Verification items for this drawing (mm, ordinates from the low corner). A direction names the side the tool comes from. Round coordinates to 2 decimals unless told otherwise and drop trailing zeros. Write each loop counter-clockwise with the first axis right and the second up, starting at its lowest first coordinate (ties: lowest second). Pieces come first, ordered by that corner, then holes. Notation, with made-up numbers: M 72,3.5 L 98,3.5 A31 cw 98,41.5 Z; hole C 57.5,3.5 d1. An arc over 180 degrees is marked long. One line per question, with ' | ' between items. Start each with the question number.
Q1. Tool access check on the marked faces 1, 2 and 3. Record the directions out of +Z, -Z, +X, -X, +Y, -Y that give a thin tool (end or side, any length) a straight path to the whole face; none if there is none.
Q2. Gauge pin test, flat ends, axial feed: pin 1 (3 mm diameter, centred on x = 41, y = 21, fed in from -Z); pin 2 (5 mm diameter, centred on x = 32.5, z = 35, fed in from -Y); pin 3 (12 mm diameter, centred on y = 32, z = 68, fed in from -X) (1 decimal). Record the tip position at first contact, or that the pin passes through.
Q3. Cross-section at B-B (y = 29). Record the boundary of the cut face in (x, z) (1 decimal).
Q4. Thickness scan on line 1 along X through (y, z) = (32, 61.5) (1 decimal); line 2 along Y through (x, z) = (65.5, 50.5); line 3 along X through (y, z) = (10.5, 40) (1 decimal). Record the ranges inside material, lowest first. Write a range as from..to.
Q5. Cross-section at A-A (y = 24). Record the boundary of the cut face in (x, z) (1 decimal).
Q6. Release check for a two-part mould opening along Z. For the marked faces 4, 5, 6 and 7 record: released by +Z, released by -Z, zero draft, split by the parting line, or undercut.
Q7. Cross-section at C-C (y = 4.5). Record the boundary of the cut face in (x, z), then the cut area to 3 significant figures.
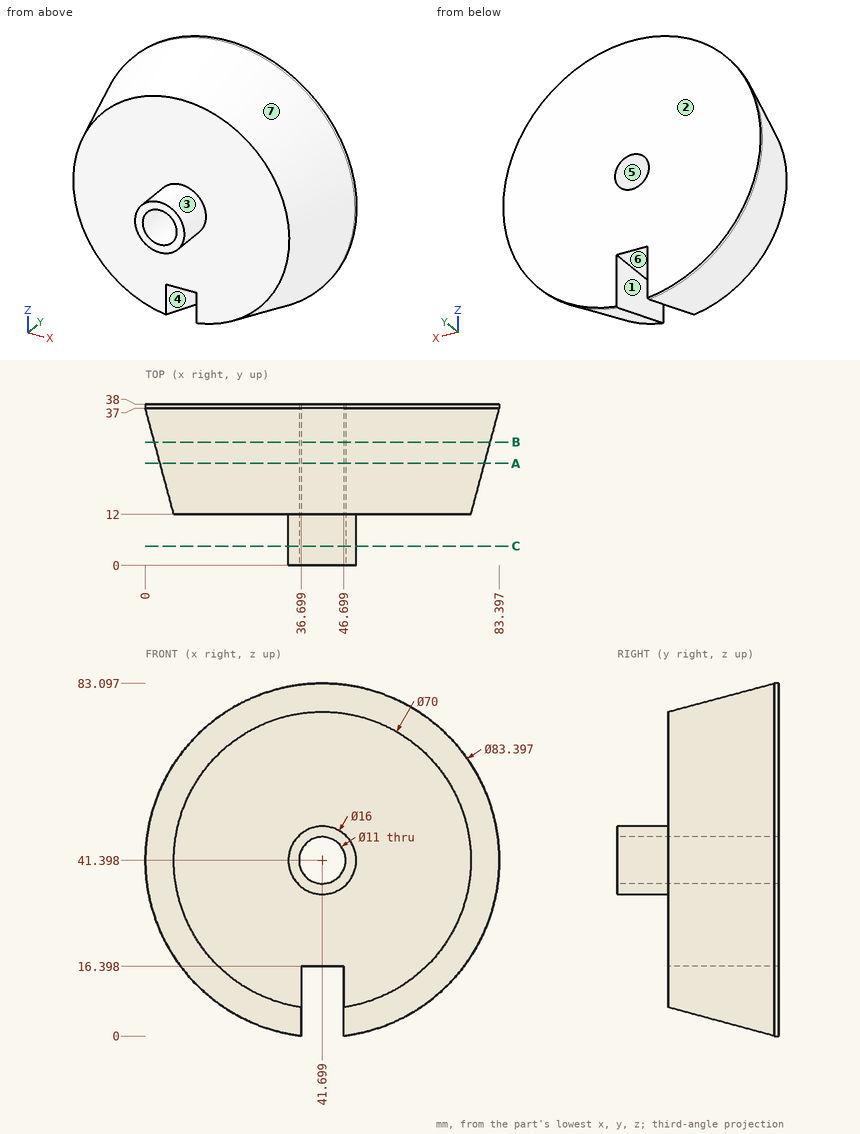
Determined:
1) face 1: -Z, +Y, -Y | face 2: +Z, -Z, +X, -X, +Y | face 3: -Y
2) pin 1: stops at z = 16.4 | pin 2: stops at y = 12 | pin 3: stops at x = 6.5
3) outline: M 36.7,2.2 L 36.7,16.4 L 46.7,16.4 L 46.7,2.2 A39.6 ccw long Z; hole C 41.7,41.4 d11
4) line 1: x = 6.7..76.7 | line 2: y = 12..38 | line 3: x = 33.8..36.4, 47..49.6
5) outline: M 36.7,3.5 L 36.7,16.4 L 46.7,16.4 L 46.7,3.5 A38.2 ccw long Z; hole C 41.7,41.4 d11
6) face 4: zero draft | face 5: undercut | face 6: released by -Z | face 7: split by the parting line
7) outline: C 41.7,41.4 d16; hole C 41.7,41.4 d11 | area: 106 mm²
